Could you check a few things on this drawing? It's one solid part, dimensions in mm from its lowest x, y, z. Give positions to 0.01 mm unless a question says otherwise; leave off trailing zeros. Write each loop counter-clockwise with the first axis right and the second up, starting at its lowest first coordinate (ties: lowest second). Pieces come first, ordered by that corner, then holes.
1. Suppose I cut it at A-A (x = 147.5). Please give me the cut outline in (y, z), and give its area (3 significant figures).
2. If I drill on probe 1 along X at (y, z) = (1.9, 8); probe 2 along X at (y, z) = (1.1, 27); probe 3 along Z at (x, y) = (19, 2.2), over which ranges is the centre line in solid material (lowest first)?
3. I'm going to push flat-ended pins straight in: pin 1 (1.5 mm diameter, centred on x = 341.5, y = 1, fed in from -Z); pin 2 (1.5 mm diameter, centred on y = 1.5, z = 49, fed in from +X); pin 3 (0.9 mm diameter, centred on x = 21.5, y = 2, fed in from +Z). Where does each tip first touch, or does it pass through?
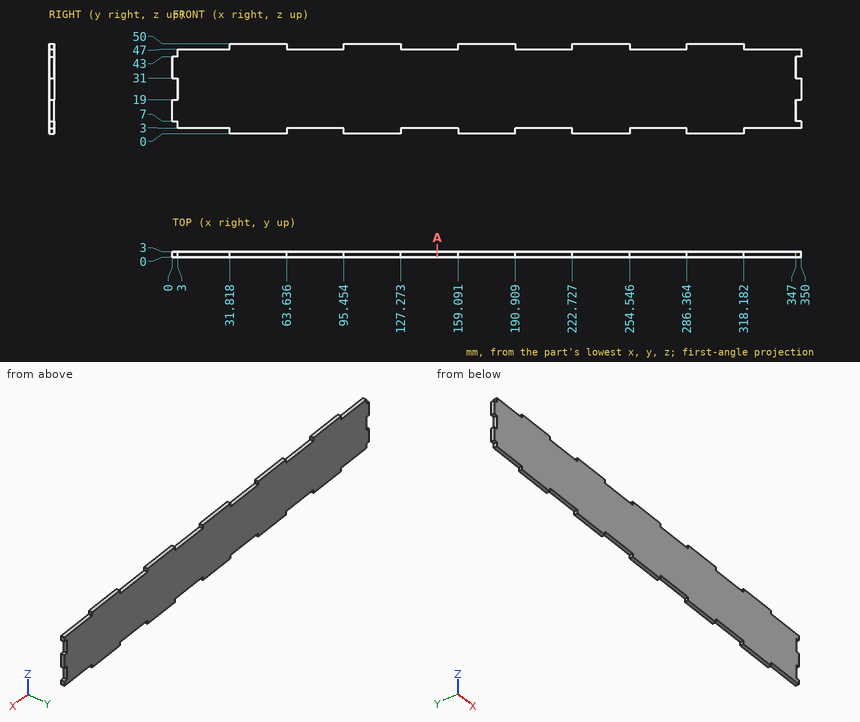
Checks:
1. outline: (0, 3) - (3, 3) - (3, 47) - (0, 47) - close
1. area: 132 mm2
2. probe 1: x = 0 to 347
2. probe 2: x = 3 to 350
2. probe 3: z = 3 to 47
3. pin 1: stops at z = 3
3. pin 2: stops at x = 318.18
3. pin 3: stops at z = 47
